Can you work these out from the model? Positions are in its coordinate system, mm. A direction names the side the tool comes from. Give positions to 0.01 mm unless a question says otherwise; leave off trailing zeros. Loops run counter-clockwise (first coordinate to the right, second up) from the corner with the lowest first, then second, coordinate; pieces in that order, holes last. Notation, with made-up numbers: (-10, -3) - (30, -3) arc R26 ccw to (30, 16) - close; hole circle Ø10 at (69, -16). An arc over 180 degrees is marked (long way). Answer in a Markdown table with one row per item.
Autodesk Inventor part; units mm, degrees
ref_plane "Work Plane1" through (0, 0, 5.5) normal (0, 0, 1) x (1, 0, 0)
ref_plane "YZ Plane" through (0, 0, 0) normal (1, 0, 0) x (0, 1, 0)
ref_plane "XZ Plane" through (0, 0, 0) normal (0, 1, 0) x (-1, 0, 0)
sketch "Sketch1" plane through (0, 0, 0) normal (1, 0, 0) x (0, 1, 0)
  circle A0 centre (0, 0) radius 4
  dimension "d0" = 8
extrude "Extrusion1" add sketch "Sketch1" along normal blind 52
chamfer "Chamfer1" distance 0.5 angle 45 2 edges at (0, -4, 0) (52, -4, 0)
ref_plane "Work Plane1" through (0, 0, 5.5) normal (0, 0, 1) x (1, 0, 0)
sketch "Sketch2" plane through (0, 0, 5.5) normal (0, 0, 1) x (1, 0, 0)
  line L0 (0, 0) -> (3.5, 0) construction
  circle A0 centre (3.5, 0) radius 1.25
  dimension "d7" = 3.5
  dimension "d8" = 2.5
extrude "Extrusion2" cut sketch "Sketch2" against normal blind 52
sketch "Sketch3" plane through (0, 0, 5.5) normal (0, 0, 1) x (1, 0, 0)
  line L0 (52, 3.5) -> (52, -3.5) construction
  line L1 (52, 0) -> (52, 3) construction
  line L2 (52, 3) -> (44, 3) construction
  line L3 (44, 3) -> (44, 4) construction
  line L4 (0.5, 4) -> (51.5, 4) construction
  line L5 (44, 4) -> (52, 4)
  line L6 (52, 4) -> (52, 3)
  line L7 (52, 3) -> (44, 3)
  line L8 (44, 3) -> (44, 4)
  point P0 (0, 0)
  dimension "d11" = 3
  dimension "d12" = 8
extrude "Extrusion3" cut sketch "Sketch3" against normal blind 52
properties part number "Crankshaft outer rod" material "Steel, Alloy"
Q1. Imagine slicing it at D-D, the plane x = 21.5. Write out the boundary of the cut face in (y, z).
Checked values:
| item | result |
|---|---|
| outline | circle Ø8 at (0, 0) |
Q2. Imagine slicing it at C-C, the plane x = 3.5. Write out the boundary of the cut face in (y, z).
Checked values:
| item | result |
|---|---|
| outline | (-1.25, -3.8) - (-1.25, 3.8) arc R4 ccw to start; (1.25, -3.8) arc R4 ccw to (1.25, 3.8) - close |
Q3. If I drill on line 1 (X direction, y = 0, z = 1.75); line 2 (Y direction, x = 3.5, z = 0); line 3 (Y direction, x = 3.5, z = -0.75), over which ranges is the centre line in solid material (lowest first)? Write a range as [from, to].
Checked values:
| item | result |
|---|---|
| line 1 | x = [0, 2.25], [4.75, 52] |
| line 2 | y = [-4, -1.25], [1.25, 4] |
| line 3 | y = [-3.93, -1.25], [1.25, 3.93] |
Q4. Imagine slicing it at B-B, the plane z = 0. Write out the boundary of the cut face in (x, y), and give its area (3 significant figures).
Checked values:
| item | result |
|---|---|
| outline | (0, -3.5) - (0.5, -4) - (51.5, -4) - (52, -3.5) - (52, 3) - (44, 3) - (44, 4) - (0.5, 4) - (0, 3.5) - close; hole circle Ø2.5 at (3.5, 0) |
| area | 403 mm² |
Q5. If we mould it in two halves opening along Y, with no side actions, what happens to faces 1 (the face through (4.69, 0.38, 0.06)), 2 (the face through (51.86, -3.64, -0.13)), 3 (the face through (52, 0, 0))? For each: released by +Y, released by -Y, zero draft, split by the parting line, or undercut.
Checked values:
| item | result |
|---|---|
| face 1 | undercut |
| face 2 | split by the parting line |
| face 3 | zero draft |
Q6. Imagine slicing it at A-A, the plane y = 0. Write out the boundary of the cut face in (x, z), and give its area (4 significant figures).
Checked values:
| item | result |
|---|---|
| outline | (0, -3.5) - (0.5, -4) - (2.25, -4) - (2.25, 4) - (0.5, 4) - (0, 3.5) - close; (4.75, -4) - (51.5, -4) - (52, -3.5) - (52, 3.5) - (51.5, 4) - (4.75, 4) - close |
| area | 395.5 mm² |
Q7. For pin 1 (3 mm diameter, centred on x = 26, y = -2, fed in from -Z); pin 2 (1 mm diameter, centred on y = 2.5, z = 0, fed in from -X); pin 3 (3 mm diameter, centred on x = 24, y = -2.5, fed in from +Z); pin 4 (4 mm diameter, centred on x = 47.5, z = 0.5, fed in from +Y), each with a flat end and sliding along its axis, tell me the tip position at first contact or that it passes through.
Checked values:
| item | result |
|---|---|
| pin 1 | stops at z = -3.97 |
| pin 2 | stops at x = 0 |
| pin 3 | stops at z = 3.87 |
| pin 4 | stops at y = 3 |
Q8. On a 3-axis mill with a long thin cutter (end or side, diameter ignored), from which of +Z, -Z, +X, -X, +Y, -Y can I reach the whole of each face in a straight line? I mean faces 4 (the face through (0, 0, 0)), 5 (the face through (44, 3.4, 0)). Say none if no direction works.
Checked values:
| item | result |
|---|---|
| face 4 | +Z, -Z, -X, +Y, -Y |
| face 5 | +Z, -Z, +X, +Y |
